Build history of the part. All positions in model axes, mm. A direction names the side the tool comes from. Round coordinates to 2 decimals unless told otherwise and drop trailing zeros. Loops run counter-clockwise (first coordinate to the right, second up) from the corner with the lowest first, then second, coordinate; pieces in that order, holes last.
from build123d import *

# Parameters (mm, degrees)
SKETCH1_W           = 30
SKETCH1_H           = 30
BOSS_EXTRUDE1_DEPTH = 30
SKETCH2_W           = 45
SKETCH2_H           = 45
BOSS_EXTRUDE2_DEPTH = 10
SKETCH4_W           = 45
SKETCH4_H           = 45
BOSS_EXTRUDE3_DEPTH = 20
SKETCH5_R           = 9.5
CUT_EXTRUDE1_DEPTH  = 40
SKETCH6_W           = 26
SKETCH6_H           = 26
CUT_EXTRUDE2_DEPTH  = 30
SKETCH7_R           = 2.5
CUT_EXTRUDE3_DEPTH  = 20


with BuildPart() as part:
    # Sketch1 → Boss-Extrude1 (new body)
    with BuildSketch(Plane(origin=(0, 0, 0), x_dir=(1, 0, 0), z_dir=(0, 1, 0))):
        with Locations((15, 15)):
            Rectangle(SKETCH1_W, SKETCH1_H)
    extrude(amount=BOSS_EXTRUDE1_DEPTH)

    # Sketch2 → Boss-Extrude2 (add)
    with BuildSketch(Plane(origin=(0, 30, 0), x_dir=(1, 0, 0), z_dir=(0, 1, 0))):
        with Locations((15, 15)):
            Rectangle(SKETCH2_W, SKETCH2_H)
    extrude(amount=BOSS_EXTRUDE2_DEPTH)

    # Sketch4 → Boss-Extrude3 (add)
    with BuildSketch(Plane(origin=(0, 40, 0), x_dir=(1, 0, 0), z_dir=(0, 1, 0))):
        with Locations((15, 15)):
            Rectangle(SKETCH4_W, SKETCH4_H)
    extrude(amount=BOSS_EXTRUDE3_DEPTH)

    # Sketch5 → Cut-Extrude1 (cut)
    with BuildSketch(Plane(origin=(0, 60, 0), x_dir=(1, 0, 0), z_dir=(0, 1, 0))):
        with Locations((15, 15)):
            Circle(SKETCH5_R)
    extrude(amount=-CUT_EXTRUDE1_DEPTH, mode=Mode.SUBTRACT)

    # Sketch6 → Cut-Extrude2 (cut)
    with BuildSketch(Plane(origin=(0, 60, 0), x_dir=(1, 0, 0), z_dir=(0, 1, 0))):
        with Locations((15, 15)):
            Rectangle(SKETCH6_W, SKETCH6_H)
    extrude(amount=-CUT_EXTRUDE2_DEPTH, mode=Mode.SUBTRACT)

    # Sketch7 → Cut-Extrude3 (cut)
    with BuildSketch(Plane.XZ):
        with Locations((25, -25)):
            Circle(SKETCH7_R)
        with Locations((5, -25)):
            Circle(SKETCH7_R)
        with Locations((5, -5)):
            Circle(SKETCH7_R)
        with Locations((25, -5)):
            Circle(SKETCH7_R)
    extrude(amount=-CUT_EXTRUDE3_DEPTH, mode=Mode.SUBTRACT)


solid = part.part
(1) Probe line 1 (Z direction, x = 25, y = 12.5); line 2 (Z direction, x = 18, y = 45.5); line 3 (X direction, y = 36, z = -16.5). List the from-to ranges inside material, lowest first.
Responses:
line 1: z = -30 to -27.5, -22.5 to -7.5, -2.5 to 0
line 2: z = -37.5 to -28, -2 to 7.5
line 3: x = -7.5 to 2, 28 to 37.5
(2) Slice it at C-C on x = 15. List the corners of the cut face in (y, z), plus the area to 3 significant figures.
Responses:
outline: (0, -30) - (30, -30) - (30, -37.5) - (60, -37.5) - (60, -28) - (30, -28) - (30, -24.5) - (20, -24.5) - (20, -5.5) - (30, -5.5) - (30, -2) - (60, -2) - (60, 7.5) - (30, 7.5) - (30, 0) - (0, 0) - close
area: 1,280 mm2
(3) Which spindle directions (+Z, -Z, +X, -X, +Y, -Y) get a long thin tool onto all of the face, cutting with end or side? Do faces 4 (the face through (5.51, 25.07, -15.42)), 5 (the face through (30, 15, -15)), 6 (the face through (15, 15, -30)), 7 (the face through (5, 20, -25)), 8 (the face through (15, 60, -30)). Say none if no direction does.
Responses:
face 4: +Y
face 5: +Z, -Z, +X, -Y
face 6: -Z, +X, -X, -Y
face 7: -Y
face 8: +Z, -Z, +X, -X, +Y
(4) Slice it at B-B on z = -15. List the corners of the cut face in (x, y).
Responses:
outline: (-7.5, 30) - (0, 30) - (0, 0) - (30, 0) - (30, 30) - (37.5, 30) - (37.5, 60) - (28, 60) - (28, 30) - (24.5, 30) - (24.5, 20) - (5.5, 20) - (5.5, 30) - (2, 30) - (2, 60) - (-7.5, 60) - close
(5) Pin check, flat tips, straight feed: P1, Ø1, axis at y = 10, z = -3.5, coming from the +X side; P2, Ø1.5, axis at x = 6, z = -6, coming from the -Y side; P3, Ø3, axis at x = 5, z = -5, coming from the +Y side. Stop position of each tip, or through.
Responses:
P1: stops at x = 30
P2: stops at y = 20
P3: stops at y = 30
(6) Slice it at A-A on y = 39. List the corners of the cut face in (x, z), plus the area to 3 significant figures.
Responses:
outline: (-7.5, -37.5) - (37.5, -37.5) - (37.5, 7.5) - (-7.5, 7.5) - close; hole (2, -28) - (28, -28) - (28, -2) - (2, -2) - close
area: 1,350 mm2
(7) Pull direction X, two halves, no side cores. Call faces 1 (the face through (15, 15, 0)), 2 (the face through (0, 15, -15)), 3 (the face through (15, 45, -28)): +X half, -X half, draft (parallel to the pull), parting line (faces both ways), or undercut.
Responses:
face 1: draft
face 2: -X half
face 3: undercut
(8) Slice it at D-D on y = 27. List the corners of the cut face in (x, z), plus the area to 3 significant figures.
Responses:
outline: (0, -30) - (30, -30) - (30, 0) - (0, 0) - close; hole circle Ø19 at (15, -15)
area: 616 mm2
